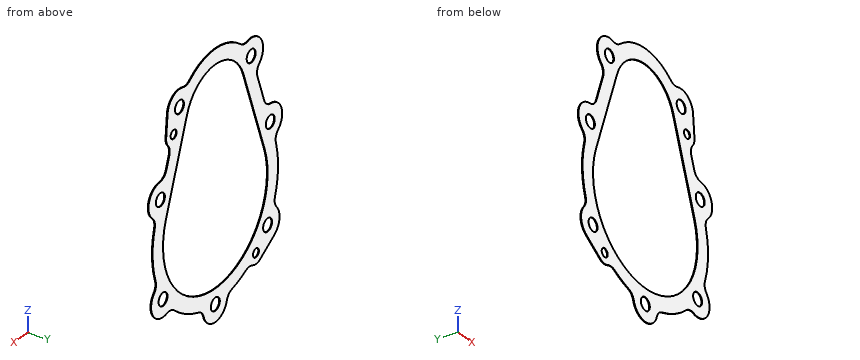
from build123d import *

# Parameters (mm, degrees)
F0_R     = 3
F0_R_2   = 2
F1_DEPTH = 0.3


with BuildPart() as f1:
    # F0 (on Front) → F1 (new body)
    with BuildSketch(Plane.XZ):
        with BuildLine():
            ThreePointArc((21.670889, 20.022763), (19.250386, 19.900136), (17.05657, 20.930204))
            ThreePointArc((17.05657, 20.930204), (0, 27), (-17.05657, 20.930204))
            ThreePointArc((-17.05657, 20.930204), (-19.250386, 19.900136), (-21.670889, 20.022763))
            ThreePointArc((-21.670889, 20.022763), (-30.920732, 16.38223), (-29.485281, 6.545942))
            ThreePointArc((-29.485281, 6.545942), (-28.0542, 4.083792), (-28.199536, 1.239666))
            Line((-28.199536, 1.239666), (-32.769553, -11.686292))
            ThreePointArc((-32.769553, -11.686292), (-34.485775, -14.021257), (-37.208965, -15.012077))
            ThreePointArc((-37.208965, -15.012077), (-44.32696, -20.375958), (-42.064669, -28.996811))
            ThreePointArc((-42.064669, -28.996811), (-40.585524, -31.306286), (-40.547083, -34.04856))
            ThreePointArc((-40.547083, -34.04856), (-41.986361, -46.070271), (-39.936462, -58.003039))
            ThreePointArc((-39.936462, -58.003039), (-39.797967, -60.58066), (-40.963571, -62.883848))
            ThreePointArc((-40.963571, -62.883848), (-42.935234, -69.23228), (-39.427861, -74.879259))
            Line((-39.427861, -74.879259), (-29.970354, -81.164303))
            ThreePointArc((-29.970354, -81.164303), (-27.561454, -81.98713), (-25.05963, -81.517324))
            ThreePointArc((-25.05963, -81.517324), (-22.750585, -81.037396), (-20.478412, -81.66926))
            ThreePointArc((-20.478412, -81.66926), (-15.972467, -83.844308), (-11.239844, -85.468085))
            ThreePointArc((-11.239844, -85.468085), (-9.01527, -86.777506), (-7.740259, -89.021978))
            ThreePointArc((-7.740259, -89.021978), (0, -95), (7.740259, -89.021978))
            ThreePointArc((7.740259, -89.021978), (9.01527, -86.777506), (11.239844, -85.468085))
            ThreePointArc((11.239844, -85.468085), (19.86092, -82.007349), (27.510347, -76.736112))
            ThreePointArc((27.510347, -76.736112), (29.83121, -75.606111), (32.406393, -75.78428))
            ThreePointArc((32.406393, -75.78428), (41.666667, -72.63854), (40.963571, -62.883848))
            ThreePointArc((40.963571, -62.883848), (39.797967, -60.58066), (39.936462, -58.003039))
            ThreePointArc((39.936462, -58.003039), (41.986361, -46.070271), (40.547083, -34.04856))
            ThreePointArc((40.547083, -34.04856), (40.585524, -31.306286), (42.064669, -28.996811))
            ThreePointArc((42.064669, -28.996811), (44.32696, -20.375958), (37.208965, -15.012077))
            ThreePointArc((37.208965, -15.012077), (34.485775, -14.021257), (32.769553, -11.686292))
            Line((32.769553, -11.686292), (30.817469, -6.164966))
            ThreePointArc((30.817469, -6.164966), (30.615698, -3.584652), (31.731116, -1.24915))
            ThreePointArc((31.731116, -1.24915), (32.693172, 0.477163), (32.911198, 2.441385))
            Line((32.911198, 2.441385), (31.968768, 13.075533))
            ThreePointArc((31.968768, 13.075533), (28.474085, 19.001252), (21.670889, 20.022763))
        make_face()
        with Locations((-35, -68.216374)):
            Circle(F0_R, mode=Mode.SUBTRACT)
        with Locations((-27.202941, -77)):
            Circle(F0_R_2, mode=Mode.SUBTRACT)
        with Locations((0, -87)):
            Circle(F0_R, mode=Mode.SUBTRACT)
        with Locations((35, -68.216374)):
            Circle(F0_R, mode=Mode.SUBTRACT)
        with Locations((-36.769553, -23)):
            Circle(F0_R, mode=Mode.SUBTRACT)
        with Locations((-24, 12.369317)):
            Circle(F0_R, mode=Mode.SUBTRACT)
        with BuildLine():
            Line((-32.998316, -33.333333), (-18.856181, 6.666667))
            ThreePointArc((-18.856181, 6.666667), (0, 20), (18.856181, 6.666667))
            Line((18.856181, 6.666667), (32.998316, -33.333333))
            ThreePointArc((32.998316, -33.333333), (0, -80), (-32.998316, -33.333333))
        make_face(mode=Mode.SUBTRACT)
        with Locations((36.769553, -23)):
            Circle(F0_R, mode=Mode.SUBTRACT)
        with Locations((27.930718, 2)):
            Circle(F0_R_2, mode=Mode.SUBTRACT)
        with Locations((24, 12.369317)):
            Circle(F0_R, mode=Mode.SUBTRACT)
    extrude(amount=F1_DEPTH)


solid = f1.part
The model under review builds one solid part; all positions refer to its coordinate system, in mm. Round coordinates to 2 decimals unless told otherwise and drop trailing zeros. Order: outer loops, then holes, each group sorted by start corner. A loop starts at its lowest first (then second) coordinate and runs counter-clockwise, first axis right, second up. Notation, with made-up numbers: (-9.75, -33) -> (28.25, -33) arc R28 ccw to (28.25, 6) -> close; hole circle Ø8 at (0.25, -25.5). An arc over 180 degrees is marked (long way). Use CSV: the item, a comma, the result in double quotes. Start each with the question number.
(1) Consider section B-B on x = 0. Write out the cut boundary in (y, z), and give its area (3 significant figures).
(2) Consider section A-A on z = -45. Write out the cut boundary in (x, y).
(3) Consider section D-D on x = -14. Write out the cut boundary in (y, z).
(4) Consider section C-C on z = -67. Write out the cut boundary in (x, y).
(5) Insertion check: pin 1 (3.5 mm diameter, centred on x = 24, z = 12.37, fed in from -Y). The pin has a flat end and moves straight along its axis. Give the tip position at first contact, or say it passes through.
(6) Wall thickness on probe 1 along X at (y, z) = (-0.1, -44.5); probe 2 along X at (y, z) = (-0.05, -76.5); probe 3 along Z at (x, y) = (-37, -0.2): over which ranges is each line inside the solid? List them lowest first. Write a range as from..to.
Responses:
1,outline,"(-0.3, -95) -> (0, -95) -> (0, -90) -> (-0.3, -90) -> close; (-0.3, -84) -> (0, -84) -> (0, -80) -> (-0.3, -80) -> close; (-0.3, 20) -> (0, 20) -> (0, 27) -> (-0.3, 27) -> close"
1,area,"4.80 mm²"
2,outline,"(-42, -0.3) -> (-35, -0.3) -> (-35, 0) -> (-42, 0) -> close; (35, -0.3) -> (42, -0.3) -> (42, 0) -> (35, 0) -> close"
3,outline,"(-0.3, -84.6) -> (0, -84.6) -> (0, -77.08) -> (-0.3, -77.08) -> close; (-0.3, 14.28) -> (0, 14.28) -> (0, 23.09) -> (-0.3, 23.09) -> close"
4,outline,"(-42.91, -0.3) -> (-37.74, -0.3) -> (-37.74, 0) -> (-42.91, 0) -> close; (-32.26, -0.3) -> (-27.22, -0.3) -> (-27.22, 0) -> (-32.26, 0) -> close; (27.22, -0.3) -> (32.26, -0.3) -> (32.26, 0) -> (27.22, 0) -> close; (37.74, -0.3) -> (42.91, -0.3) -> (42.91, 0) -> (37.74, 0) -> close"
5,pin 1,"through"
6,probe 1,"-42..-35, 35..42"
6,probe 2,"-36.99..-29.14, -25.27..-15.26, 15.26..27.8"
6,probe 3,"-76.49..-70.45, -65.98..-25.99, -20.01..-15"
